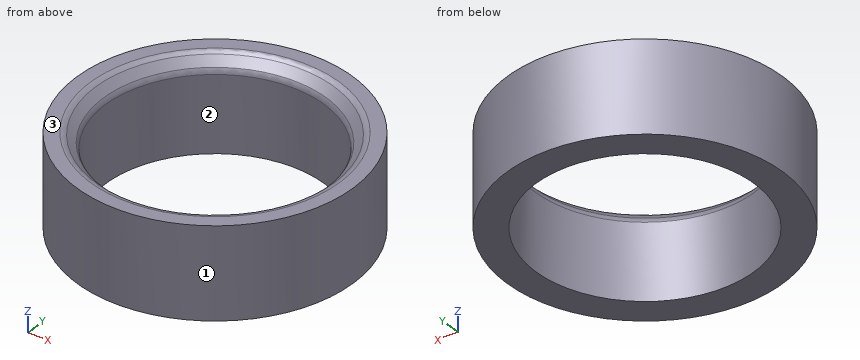
from build123d import *

# Parameters (mm, degrees)
F2_R = 1.5
F3_R = 1.5


with BuildPart() as f1:
    # F0 (on Front) → F1 (revolve)
    with BuildSketch(Plane.XZ):
        Polygon((21.6, 15.6), (21.6, 0), (27.3, 0), (27.3, 18), (24, 18), align=None)
    revolve(axis=Axis((0, 0, 4.861747), (0, 0, -1)))

    # F2
    f2_edges = [f1.edges().sort_by_distance(p)[0] for p in [
        (-21.6, 0, 15.6),
    ]]
    fillet(f2_edges, radius=F2_R)

    # F3
    f3_edges = [f1.edges().sort_by_distance(p)[0] for p in [
        (-24, 0, 18),
    ]]
    fillet(f3_edges, radius=F3_R)


solid = f1.part
Source: CAD feature listing. Evaluate the final solid. Frame: model axes, mm. Face numbers are marked on the shaded views. Coordinates: 2 decimals unless noted, no trailing zeros. Order: outer loops, then holes, each group sorted by start corner. A loop starts at its lowest first (then second) coordinate and runs counter-clockwise, first axis right, second up. Notation, with made-up numbers: M 66.25,53 L 124.25,53 A26 ccw 124.25,71 Z; hole C -19.75,56.25 d8. An arc over 180 degrees is marked long. Write each question's results on one line, items separated by ' | '. Start each with the question number.
1. Section A-A, the plane z = 9.75. Return the cut outline in (x, y).
2. Pin query (flat end, axial travel): pin 1 (4 mm diameter, centred on x = -4, z = 13.5, fed in from +Y); pin 2 (5 mm diameter, centred on y = -15, z = 10.5, fed in from -X); pin 3 (6 mm diameter, centred on x = 15.5, z = 14, fed in from -Y). Return the tip coordinate at first contact, or that it passes through.
3. Material intervals for L1, parallel to Y at x = 0, z = 3.5; L2, parallel to Y at x = -12, z = 6.25, sorted ascending.
4. Draft query along X for the marked faces 1, 2 and 3. Return one class per face: +X half, -X half, draft (parallel to the pull), parting line (faces both ways), or undercut.
Solution:
1) outline: C 0,0 d54.6; hole C 0,0 d43.2
2) pin 1: y = 27.23 | pin 2: x = -24.27 | pin 3: y = -24.27
3) L1: -27.3 to -21.6, 21.6 to 27.3 | L2: -24.52 to -17.96, 17.96 to 24.52
4) face 1: parting line | face 2: undercut | face 3: draft
